For this review, use the dimensioned drawing (mm, ordinates from the lowest corner) and the shaded views. A direction names the side the tool comes from. Coordinates: 2 decimals unless noted, no trailing zeros. Loops run counter-clockwise (first coordinate to the right, second up) from the corner with the lowest first, then second, coordinate; pieces in that order, holes last.
1. Mouldability with a two-part tool opening along Y and no side actions: class the marked faces 3, 4 and 5 as pulls with the +Y half, pulls with the -Y half, needs draft (parallel to the pull), parting line crosses it, or undercut.
2. Machinability: for the marked faces 1 and 2, which of the approach directions +Z, -Z, +X, -X, +Y, -Y give a long, thin tool a straight path to every point of the face, cutting with its end or side? Answer none if there is none.
3. Clearance check with flat-ended pins moving along their axes: P1, Ø3, axis at y = 33, z = 7, coming from the +X side; P2, Ø1, axis at y = 39.5, z = 4.5, coming from the +X side; P3, Ø2, axis at y = 28.5, z = 6, coming from the -X side. State where each tip first meets the part, or that it passes through.
4. To check wall thickness, follow probe 1 along Y at (x, z) = (32, 3.5); probe 2 along Y at (x, z) = (32, 3); probe 3 along X at (y, z) = (36.5, 3). State the ranges of each line that lie inside material, in increasing order.
5. Take a section at C-C, the plane z = 7. State the section outline as (x, y) points, then the cut area to 3 significant figures.
6. Take a section at A-A, the plane x = 32. State the section outline as (y, z) points.
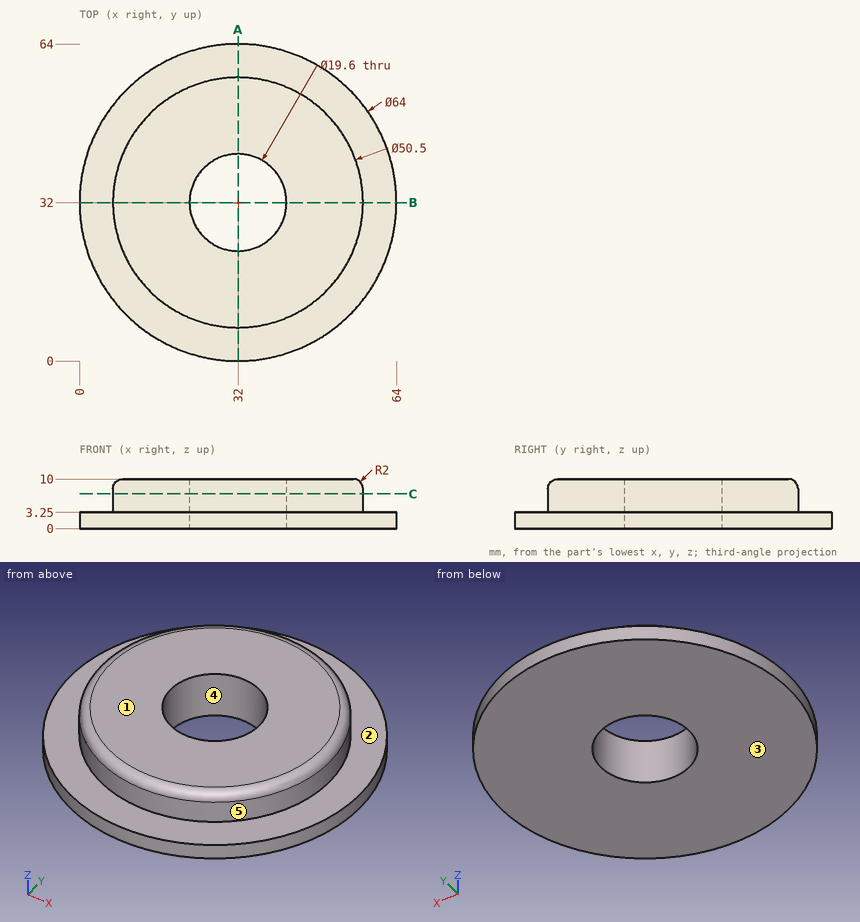
Results list:
1. face 3: needs draft
1. face 4: undercut
1. face 5: parting line crosses it
2. face 1: +Z, +X, -X, +Y, -Y
2. face 2: +Z
3. P1: stops at x = 57.25
3. P2: stops at x = 56.26
3. P3: stops at x = 6.87
4. probe 1: y = 6.75 to 22.2, 41.8 to 57.25
4. probe 2: y = 0 to 22.2, 41.8 to 64
4. probe 3: x = 0.32 to 23.29, 40.71 to 63.68
5. outline: circle Ø50.5 at (32, 32); hole circle Ø19.6 at (32, 32)
5. area: 1,700 mm2
6. outline: (0, 0) - (22.2, 0) - (22.2, 10) - (8.75, 10) arc R2 ccw to (6.75, 8) - (6.75, 3.25) - (0, 3.25) - close; (41.8, 0) - (64, 0) - (64, 3.25) - (57.25, 3.25) - (57.25, 8) arc R2 ccw to (55.25, 10) - (41.8, 10) - close
